Geometry: final body of the model. Coordinates: model frame, mm. Round coordinates to 2 decimals unless told otherwise and drop trailing zeros. Write each loop counter-clockwise with the first axis right and the second up, starting at its lowest first coordinate (ties: lowest second). Pieces come first, ordered by that corner, then holes.
from build123d import *

# Parameters (mm, degrees)
SKETCH1_W           = 135.25
SKETCH1_H           = 12.42
BOSS_EXTRUDE1_DEPTH = 4
CUT_EXTRUDE1_DEPTH  = 156.797364869
CUT_EXTRUDE2_DEPTH  = 2.3
FILLET1_R           = 5
FILLET2_R           = 2


with BuildPart() as part:
    # Sketch1 → Boss-Extrude1 (new body)
    with BuildSketch(Plane(origin=(0, 0, 0), x_dir=(0, 0, -1), z_dir=(1, 0, 0))):
        with Locations((67.625, 6.21)):
            Rectangle(SKETCH1_W, SKETCH1_H)
        Polygon((148.25, 0), (135.25, 0), (135.25, 12.42), (148.25, 12.42), (155.25, 6.21), align=None)
    extrude(amount=BOSS_EXTRUDE1_DEPTH)

    # Sketch7 → Cut-Extrude1 (cut, through all)
    with BuildSketch(Plane.ZY):
        with BuildLine():
            ThreePointArc((-2.27, 6.21), (-3.168108515, 8.592801832), (-5.415564859, 9.79))
            Line((-5.415564859, 9.79), (-6.76734979, 9.709244254))
            ThreePointArc((-6.76734979, 9.709244254), (-9.49, 6.21), (-6.76734979, 2.710755746))
            Line((-6.76734979, 2.710755746), (-5.415564859, 2.63))
            ThreePointArc((-5.415564859, 2.63), (-3.168108515, 3.827198168), (-2.27, 6.21))
        make_face()
    extrude(amount=-CUT_EXTRUDE1_DEPTH, mode=Mode.SUBTRACT)

    # Sketch7<3> → Cut-Extrude2 (cut)
    with BuildSketch(Plane.ZY):
        with BuildLine():
            ThreePointArc((-6.76734979, 2.710755746), (-9.49, 6.21), (-6.76734979, 9.709244254))
            Line((-6.76734979, 9.709244254), (-23.410182873, 8.715))
            ThreePointArc((-23.410182873, 8.715), (-25.77, 6.21), (-23.410182873, 3.705))
            Line((-23.410182873, 3.705), (-6.76734979, 2.710755746))
        make_face()
    extrude(amount=-CUT_EXTRUDE2_DEPTH, mode=Mode.SUBTRACT)

    # Fillet1
    fillet1_edges = [part.edges().sort_by_distance(p)[0] for p in [
        (2, 0, 0),
        (2, 12.42, 0),
    ]]
    fillet(fillet1_edges, radius=FILLET1_R)

    # Fillet2
    fillet2_edges = [part.edges().sort_by_distance(p)[0] for p in [
        (3.15, 9.709244254, -6.76734979),
        (3.15, 2.710755746, -6.76734979),
    ]]
    fillet(fillet2_edges, radius=FILLET2_R)


solid = part.part
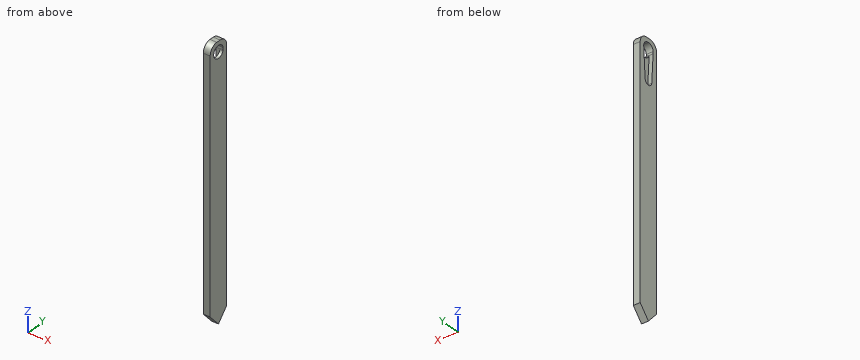
1) Line query: probe 1 along Z at (x, y) = (0.6, 7.25); probe 2 along Z at (x, y) = (1.3, 4.25); probe 3 along Y at (x, z) = (0.2, -17.5). Output: solid intervals per line, ascending.
2) Section A-A on x = 1. Output: boundary loops of the cut face in (y, z) (3 decimals).
3) Section B-B on z = -15.5. Output: boundary loops of the cut face in (x, y), plus the area to 3 significant figures.
4) First-contact query: P1, Ø5, axis at y = 1.5, z = -105.5, coming from the -X side. Flat tip, straight axial feed; report the tip coordinate or a pass-through.
Filled in:
1. probe 1: z = -154.08 to -25.54, -2.42 to 0
1. probe 2: z = -153.04 to -24.83, -2.85 to -0.06
1. probe 3: y = 0 to 3.35, 9.07 to 12.42
2. outline: (0, -148.25) - (6.21, -155.25) - (12.42, -148.25) - (12.42, -5) arc R5 ccw to (7.42, 0) - (5, 0) arc R5 ccw to (0, -5) - close; hole (2.63, -5.416) - (3.705, -23.41) arc R2.509 ccw to (8.715, -23.41) - (9.79, -5.416) arc R3.61 ccw to start
3. outline: (0, 0) - (4, 0) - (4, 12.42) - (0, 12.42) - (0, 9.19) - (2.3, 9.19) - (2.3, 3.23) - (0, 3.23) - close
3. area: 36.0 mm2
4. P1: stops at x = 0
